Part model, mm, in its own coordinate system. Coordinates: 2 decimals unless noted, no trailing zeros. Loops run counter-clockwise (first coordinate to the right, second up) from the corner with the lowest first, then second, coordinate; pieces in that order, holes last. Notation, with made-up numbers: M 87.5,-15 L 128.5,-15 A6 cw 128.5,-5 Z; hole C 23,81 d4. An arc over 180 degrees is marked long. Use a Markdown table: item, result. Add a question column.
1) Wall check: probe 1 along X at (y, z) = (-72, 0.05) (3 decimals); probe 2 along Y at (x, z) = (-50, 0.15) (3 decimals); probe 3 along Y at (x, z) = (-10, 0.1) (3 decimals). Give the ranges that are in metal, low to high. Write a range as from..to.
2) Band-saw the part on A-A (z = -0.1). State how many separate pieces and enclosed holes the cut face has, plus the area to 3 significant figures.
3) Pin check, flat tip, straight feed: pin 1 Ø1.5 at (x, y) = (-74, 22) entering from -Z. Stop position of the tip, or through.
4) Band-saw the part on B-B (y = 39.5). List the corners of the cut face in (x, z), plus the area to 3 significant figures.
from build123d import *

# Parameters (mm, degrees)
SKETCH_1_W             = 89
SKETCH_1_H             = 152
SKETCH_1_R             = 1.525
EXTRUDE_1_DEPTH        = 0.5
SKETCH_2_R             = 1.275
CUT_EXTRUDE_1_DEPTH    = 5
SKETCH_4_W             = 29
SKETCH_4_H             = 152
EXTRUDE_3_DEPTH        = 1
SKETCH_5_R             = 95
CUT_EXTRUDE_3_DEPTH    = 22
SKETCH_9_W             = 30
SKETCH_9_H             = 152
EXTRUDE_4_DEPTH        = 1
PATTERN_LINEAR_1_COUNT = 4
PATTERN_LINEAR_1_PITCH = 8
SKETCH_10_W            = 10
SKETCH_10_H            = 20
CUT_EXTRUDE_4_DEPTH    = 10
FILLET_1_R             = 2


with BuildPart() as part:
    # 草图1 → 凸台-拉伸1 (new body, symmetric)
    with BuildSketch(Plane.XY):
        with Locations((-10.5, 0)):
            Rectangle(SKETCH_1_W, SKETCH_1_H)
        with Locations((-10, 72)):
            Circle(SKETCH_1_R, mode=Mode.SUBTRACT)
        with Locations((10, 72)):
            Circle(SKETCH_1_R, mode=Mode.SUBTRACT)
        with Locations((10, -72)):
            Circle(SKETCH_1_R, mode=Mode.SUBTRACT)
        with Locations((-10, -72)):
            Circle(SKETCH_1_R, mode=Mode.SUBTRACT)
    extrude(amount=EXTRUDE_1_DEPTH, both=True)

    # 草图2 → 切除-拉伸1 (cut, symmetric)
    with BuildSketch(Plane.XY.offset(0.5)):
        with Locations((-50, 22)):
            Circle(SKETCH_2_R)
        with Locations((-50, -22)):
            Circle(SKETCH_2_R)
        with Locations((6, -33.75)):
            Circle(SKETCH_2_R)
        with Locations((6, 33.75)):
            Circle(SKETCH_2_R)
    cut_extrude_1 = extrude(amount=CUT_EXTRUDE_1_DEPTH, both=True, mode=Mode.SUBTRACT)

    # 草图4 → 凸台-拉伸3 (add)
    with BuildSketch(Plane.XY.offset(0.5)):
        with Locations((48.5, 0)):
            Rectangle(SKETCH_4_W, SKETCH_4_H)
    extrude(amount=-EXTRUDE_3_DEPTH)

    # 草图5 → 切除-拉伸3 (cut)
    with BuildSketch(Plane.XY.offset(0.5)):
        with Locations((144, 0)):
            Circle(SKETCH_5_R)
    extrude(amount=-CUT_EXTRUDE_3_DEPTH, mode=Mode.SUBTRACT)

    # 草图9 → 凸台-拉伸4 (add)
    with BuildSketch(Plane.XY.offset(0.5)):
        with Locations((-70, 0)):
            Rectangle(SKETCH_9_W, SKETCH_9_H)
    extrude(amount=-EXTRUDE_4_DEPTH)

    # 阵列(线性)1: 切除-拉伸1 ×4
    with Locations(*[(-i * PATTERN_LINEAR_1_PITCH, 0, 0) for i in range(1, PATTERN_LINEAR_1_COUNT)]):
        add(cut_extrude_1, mode=Mode.SUBTRACT)

    # 草图10 → 切除-拉伸4 (cut)
    with BuildSketch(Plane.XY.offset(0.5)):
        with Locations((-85, 0)):
            Rectangle(SKETCH_10_W, SKETCH_10_H)
    extrude(amount=-CUT_EXTRUDE_4_DEPTH, mode=Mode.SUBTRACT)

    # 圆角1
    fillet_1_edges = [part.edges().sort_by_distance(p)[0] for p in [
        (-85, 10, 0),
        (-85, -10, 0),
        (-80, 10, 0),
        (-80, -10, 0),
        (63, 76, 0),
        (63, -76, 0),
        (63, -49.638694584, 0),
        (63, 49.638694584, 0),
        (-85, -76, 0),
        (-85, 76, 0),
    ]]
    fillet(fillet_1_edges, radius=FILLET_1_R)


solid = part.part
Entries:
| question | item | result |
|---|---|---|
| 1 | probe 1 | -85..-11.525, -8.475..8.475, 11.525..63 |
| 1 | probe 2 | -76..-23.275, -20.725..20.725, 23.275..76 |
| 1 | probe 3 | -76..-73.525, -70.475..-35.025, -32.475..32.475, 35.025..70.475, 73.525..76 |
| 2 | separate pieces | 1 |
| 2 | enclosed holes | 20 |
| 2 | area | 21,300 mm2 |
| 3 | pin 1 | through |
| 4 | outline | M -85,-0.5 L 57.6,-0.5 L 57.6,0.5 L -85,0.5 Z |
| 4 | area | 143 mm2 |
